Geometry: final body of the model. Coordinates: model frame, mm. A direction names the side the tool comes from. Give positions to 0.01 mm unless a question says otherwise; leave off trailing zeros. Write each loop counter-clockwise with the first axis right and the second up, starting at its lowest first coordinate (ties: lowest second). Pieces come first, ordered by that corner, then holes. Notation, with made-up numbers: M 54.5,-8.75 L 65.5,-8.75 A26 cw 65.5,22.25 Z; hole C 44,30 d1. An arc over 180 degrees is marked long. Answer as a JSON object with one key per item and string values.
from build123d import *

# Parameters (mm, degrees)
SKETCH1_W           = 40
SKETCH1_H           = 10
BOSS_EXTRUDE1_DEPTH = 5
SKETCH2_W           = 8
SKETCH2_H           = 2.1
CUT_EXTRUDE2_DEPTH  = 41
SKETCH3_W           = 10
SKETCH3_H           = 25
BOSS_EXTRUDE2_DEPTH = 10
SKETCH4_W           = 2.25
SKETCH4_H           = 26.45
CUT_EXTRUDE3_DEPTH  = 8


with BuildPart() as part:
    # Sketch1 → Boss-Extrude1 (new body)
    with BuildSketch(Plane(origin=(0, 0, 0), x_dir=(1, 0, 0), z_dir=(0, 1, 0))):
        Rectangle(SKETCH1_W, SKETCH1_H)
    extrude(amount=BOSS_EXTRUDE1_DEPTH)

    # Sketch2 → Cut-Extrude2 (cut, through all)
    with BuildSketch(Plane(origin=(20, 0, 0), x_dir=(0, 0, -1), z_dir=(1, 0, 0))):
        with Locations((-1, 2.5)):
            Rectangle(SKETCH2_W, SKETCH2_H)
    extrude(amount=-CUT_EXTRUDE2_DEPTH, mode=Mode.SUBTRACT)

    # Sketch3 → Boss-Extrude2 (add)
    with BuildSketch(Plane(origin=(0, 0, -5), x_dir=(-1, 0, 0), z_dir=(0, 0, -1))):
        with Locations((0, 17.5)):
            Rectangle(SKETCH3_W, SKETCH3_H)
    extrude(amount=-BOSS_EXTRUDE2_DEPTH)

    # Sketch4 → Cut-Extrude3 (cut)
    with BuildSketch(Plane.XY.offset(5)):
        with Locations((-1.125, 16.775)):
            Rectangle(SKETCH4_W, SKETCH4_H)
        with Locations((1.125, 16.775)):
            Rectangle(SKETCH4_W, SKETCH4_H)
    extrude(amount=-CUT_EXTRUDE3_DEPTH, mode=Mode.SUBTRACT)


solid = part.part
1) Pull-direction query (X, two-part tool) for faces 1 (the flat face through (-5, 17, 0)), 2 (the flat face through (-13, 5, 0)), 3 (the flat face through (20, 1, 0)), 4 (the flat face through (0, 10, -3)); classes: pulls with the +X half, pulls with the -X half, needs draft (parallel to the pull), parting line crosses it, or undercut.
Geometry check:
{"face 1": "pulls with the -X half", "face 2": "needs draft", "face 3": "pulls with the +X half", "face 4": "undercut"}
2) Cut plane A-A on z = 2.5. Return loops of the section in (x, y), and give its area (3 significant figures).
Geometry check:
{"outline": "M -20,0 L 20,0 L 20,1.45 L -20,1.45 Z; M -20,3.55 L -2.25,3.55 L -2.25,30 L -5,30 L -5,5 L -20,5 Z; M 2.25,3.55 L 20,3.55 L 20,5 L 5,5 L 5,30 L 2.25,30 Z", "area": "247 mm2"}
3) Cut plane C-C on x = 8.5. Return loops of the section in (y, z), and give its area (3 significant figures).
Geometry check:
{"outline": "M 0,-5 L 5,-5 L 5,5 L 3.55,5 L 3.55,-3 L 1.45,-3 L 1.45,5 L 0,5 Z", "area": "33.2 mm2"}
4) Line query: line 1 (X direction, y = 12, z = -2.5); line 2 (Y direction, x = 17.5, z = 3). Output: solid intervals per line, ascending. Write a range as from..to.
Geometry check:
{"line 1": "x = -5..-2.25, 2.25..5", "line 2": "y = 0..1.45, 3.55..5"}
5) Cut plane B-B on y = 19. Return loops of the section in (x, z).
Geometry check:
{"outline": "M -5,-5 L 5,-5 L 5,5 L 2.25,5 L 2.25,-3 L -2.25,-3 L -2.25,5 L -5,5 Z"}
6) Set-up query: faces 5 (the flat face through (5, 17, 0)), 6 (the flat face through (-20, 1, 0)), 7 (the flat face through (0, 1.45, 1)), 8 (the flat face through (0.1, 30, -3.4)), 9 (the flat face through (-2.25, 17, 1)). Return all of +Z, -Z, +X, -X, +Y, -Y with unobstructed straight access to the full face (end or side cutting, diameter ignored); none if empty.
Geometry check:
{"face 5": "+Z, -Z, +X, +Y", "face 6": "+Z, -Z, -X, +Y, -Y", "face 7": "+Z, +X, -X", "face 8": "+Z, -Z, +X, -X, +Y", "face 9": "+Z, +Y"}
7) Contact query for flat-ended pins moving along their axis: P1, Ø2, axis at y = 23.5, z = 1.5, coming from the -X side; P2, Ø12, axis at x = -15.5, y = 12.5, coming from the +Z side; P3, Ø3, axis at x = 16, z = 1, coming from the +Y side; P4, Ø5, axis at x = -7, y = 13.5, coming from the +Z side. Output: stop coordinate, or through.
Geometry check:
{"P1": "stops at x = -5", "P2": "passes through", "P3": "stops at y = 5", "P4": "stops at z = 5"}
